from build123d import *

# Parameters (mm, degrees)
F0_W      = 40
F0_H      = 32
F1_DEPTH  = 11
F3_DEPTH  = 11
F4_R      = 8
F5_DEPTH  = 76.2
F7_DEPTH  = 11
F8_R      = 8
F9_DEPTH  = 76.2
F10_R     = 2
F11_R     = 9
F12_DEPTH = 32
F13_R     = 8
F14_DEPTH = 36.068


with BuildPart() as f1:
    # F0 (on Right) → F1 (new body)
    with BuildSketch(Plane.YZ):
        with Locations((-0.2878075466, 20.7610073336)):
            Rectangle(F0_W, F0_H)
    extrude(amount=F1_DEPTH)

    # F2 (on face) → F3 (join)
    with BuildSketch(Plane.XZ.offset(20.2878075466)):
        with BuildLine():
            Line((11, 36.7610073336), (11, 4.7610073336))
            Line((11, 4.7610073336), (36, 4.7610073336))
            ThreePointArc((36, 4.7610073336), (52, 20.7610073336), (36, 36.7610073336))
            Line((36, 36.7610073336), (11, 36.7610073336))
        make_face()
    extrude(amount=-F3_DEPTH)

    # F4 (on face) → F5 (cut)
    with BuildSketch(Plane.XZ.offset(20.2878075466)):
        with Locations((36, 20.7610073336)):
            Circle(F4_R)
    extrude(amount=-F5_DEPTH, mode=Mode.SUBTRACT)

    # F6 (on face) → F7 (join)
    with BuildSketch(Plane(origin=(0, 19.7121924534, 0), x_dir=(-1, 0, 0), z_dir=(0, 1, 0))):
        with BuildLine():
            Line((-11, 4.7610073336), (-11, 36.7610073336))
            Line((-11, 36.7610073336), (-36, 36.7610073336))
            ThreePointArc((-36, 36.7610073336), (-52, 20.7610073336), (-36, 4.7610073336))
            Line((-36, 4.7610073336), (-11, 4.7610073336))
        make_face()
    extrude(amount=-F7_DEPTH)

    # F8 (on face) → F9 (cut)
    with BuildSketch(Plane(origin=(0, 19.7121924534, 0), x_dir=(-1, 0, 0), z_dir=(0, 1, 0))):
        with Locations((-36, 20.7610073336)):
            Circle(F8_R)
    extrude(amount=-F9_DEPTH, mode=Mode.SUBTRACT)

    # F10
    f10_edges = [f1.edges().sort_by_distance(p)[0] for p in [
        (36, 14.212192, 36.761007),
        (36, 14.212192, 4.761007),
        (52, 19.712192, 20.761007),
        (52, 8.712192, 20.761007),
        (36, -14.787808, 4.761007),
        (36, -14.787808, 36.761007),
        (52, -20.287808, 20.761007),
        (52, -9.287808, 20.761007),
        (18, 19.712192, 36.761007),
        (23.5, 8.712192, 36.761007),
        (11, -0.287808, 36.761007),
        (23.5, -9.287808, 36.761007),
        (18, -20.287808, 36.761007),
        (0, -0.287808, 36.761007),
        (18, -20.287808, 4.761007),
        (23.5, -9.287808, 4.761007),
        (11, -0.287808, 4.761007),
        (23.5, 8.712192, 4.761007),
        (18, 19.712192, 4.761007),
        (0, -0.287808, 4.761007),
    ]]
    fillet(f10_edges, radius=F10_R)

    # F11 (on face) → F12 (join)
    with BuildSketch(Plane(origin=(0, 0, 0), x_dir=(0, -1, 0), z_dir=(-1, 0, 0))):
        with Locations((0, 20.7610073336)):
            Circle(F11_R)
    extrude(amount=F12_DEPTH)

    # F13 (on face) → F14 (cut)
    with BuildSketch(Plane(origin=(0, 19.7121924534, 0), x_dir=(-1, 0, 0), z_dir=(0, 1, 0))):
        with Locations((-36, 20.7610073336)):
            Circle(F13_R)
    extrude(amount=-F14_DEPTH, mode=Mode.SUBTRACT)


solid = f1.part
Geometry: final body of the model. Coordinates: model frame, mm. A direction names the side the tool comes from. Give positions to 0.01 mm unless a question says otherwise; leave off trailing zeros. Write each loop counter-clockwise with the first axis right and the second up, starting at its lowest first coordinate (ties: lowest second). Pieces come first, ordered by that corner, then holes.
(1) Cut plane A-A, the plane y = -15. Return loops of the section in (x, z).
(2) Ray query, line 1 (Y direction, x = 46.5, z = 22); line 2 (Z direction, x = 36, y = -13); line 3 (X direction, y = -12, z = 21). Return the intervals inside material, ascending.
(3) Cut plane C-C, the plane x = 37. Give the number of separate pieces and of enclosed holes in the cut face, then the cut area to 3 significant figures.
(4) Mould query, pull axis Y, two halves, no side actions, for faces 6 (the flat face through (11, 0, 21)), 7 (the cylindrical face through (18.252, -19.686, 5.331)), 8 (the cylindrical face through (0.6, -0.01, 5.33)). Classes: released by +Y, released by -Y, zero draft, split by the parting line, or undercut.
(5) Cut plane B-B, the plane y = 0. Return loops of the section in (x, z), then the cut area to 3 significant figures.
(6) First-contact query: P1, Ø3, axis at y = 15, z = 24, coming from the +X side; P2, Ø3, axis at y = 11.5, z = 24.5, coming from the +X side; P3, Ø14, axis at x = 34, z = 25, coming from the -Y side; P4, Ø1.5, axis at y = 4.5, z = 31, coming from the +X side. Flat tips, straight axial feed; report the tip coordinate or a pass-through.
(7) Access query for faces 1 (the cylindrical face through (22.3, -9.9, 36.2)), 2 (the flat face through (0, -9.5, 21)), 3 (the cylindrical face through (51.996, -14.837, 20.409)), 4 (the cylindrical face through (37, 14.3, 28.7)), 5 (the cylindrical face through (22.69, -9.86, 5.36)). Directions: +Z, -Z, +X, -X, +Y, -Y. A direction counts if a zero-diameter tool reaches every point of the face in a straight line with its end or side. Return the directions, or none.
Values follow:
1. outline: (0, 6.76) arc R2 ccw to (2, 4.76) - (36, 4.76) arc R16 ccw to (36, 36.76) - (2, 36.76) arc R2 ccw to (0, 34.76) - close; hole circle Ø16 at (36, 20.76)
2. line 1: y = -20.29 to -9.29, 8.71 to 19.71
2. line 2: z = 4.76 to 12.76, 28.76 to 36.76
2. line 3: x = 0 to 28, 44 to 52
3. separate pieces: 4
3. enclosed holes: 0
3. area: 347 mm2
4. face 6: undercut
4. face 7: released by -Y
4. face 8: zero draft
5. outline: (-32, 11.76) - (0, 11.76) - (0, 6.76) arc R2 ccw to (2, 4.76) - (9, 4.76) arc R2 ccw to (11, 6.76) - (11, 34.76) arc R2 ccw to (9, 36.76) - (2, 36.76) arc R2 ccw to (0, 34.76) - (0, 29.76) - (-32, 29.76) - close
5. area: 925 mm2
6. P1: stops at x = 51.91
6. P2: stops at x = 51.84
6. P3: stops at y = -20.29
6. P4: stops at x = 11
7. face 1: +Z, +X
7. face 2: -X
7. face 3: +X, +Y, -Y
7. face 4: +Y, -Y
7. face 5: -Z, +X
